from build123d import *

# Parameters (mm, degrees)
BOSS_EXTRUDE1_DEPTH  = 5
CUT_EXTRUDE1_DEPTH   = 10
BOSS_EXTRUDE3_START  = -3
SKETCH13_R           = 2.5
BOSS_EXTRUDE3_DEPTH  = 3
CHAMFER1_SIZE        = 2
BOSS_EXTRUDE7_DEPTH  = 17
SKETCH22_R           = 1.6
CUT_EXTRUDE4_DEPTH   = 20
CUT_EXTRUDE5_DEPTH   = 7
BOSS_EXTRUDE8_START  = -20
BOSS_EXTRUDE8_DEPTH  = 20
SKETCH26_R           = 90.5
SKETCH26_R_2         = 90
CUT_EXTRUDE6_DEPTH   = 15
BOSS_EXTRUDE9_START  = 20
BOSS_EXTRUDE9_DEPTH  = 20
BOSS_EXTRUDE11_DEPTH = 20
FILLET2_R            = 6
CUT_EXTRUDE8_DEPTH   = 5
FILLET3_R            = 5
CUT_EXTRUDE9_DEPTH   = 5
FILLET4_R            = 3
CUT_EXTRUDE11_DEPTH  = 5
FILLET5_R            = 3


# Some blends are built 0.0001 mm under size
with BuildPart() as part:
    # Sketch1 → Boss-Extrude1 (new body)
    with BuildSketch(Plane.XY):
        with BuildLine():
            Line((10, 70), (0, 70))
            Line((0, 70), (0, 40))
            ThreePointArc((0, 40), (34.641016151, 20), (34.641016151, -20))
            Line((34.641016151, -20), (50.226140717, -28.998075863))
            ThreePointArc((50.226140717, -28.998075863), (74.464134482, -30.098388714), (89.334294573, -10.926290001))
            ThreePointArc((89.334294573, -10.926290001), (70.606727842, 55.809407661), (10, 89.4427191))
            Line((10, 89.4427191), (10, 70))
        make_face()
    extrude(amount=-BOSS_EXTRUDE1_DEPTH)

    # Sketch10 → Cut-Extrude1 (cut)
    with BuildSketch(Plane.ZY):
        Polygon((-5, 70), (0, 47.166644618), (0, 70), align=None)
    extrude(amount=-CUT_EXTRUDE1_DEPTH, mode=Mode.SUBTRACT)

    # Sketch13 → Boss-Extrude3 (add)
    # profile 1 of 2: a face of its own
    with BuildSketch(Plane.XY.offset(BOSS_EXTRUDE3_START)):
        with BuildLine():
            Line((37.380217316, 94.74443559), (31.380217316, 84.352130745))
            ThreePointArc((31.380217316, 84.352130745), (45, 77.942286341), (57.36097943, 69.352130745))
            Line((57.36097943, 69.352130745), (63.36097943, 79.74443559))
            Line((63.36097943, 79.74443559), (37.380217316, 94.74443559))
        make_face()
        with Locations((40.856551784, 85.765623512)):
            Circle(SKETCH13_R, mode=Mode.SUBTRACT)
        with Locations((53.846932841, 78.265623512)):
            Circle(SKETCH13_R, mode=Mode.SUBTRACT)
    # profile 2 of 2: a face of its own
    with BuildSketch(Plane.XY.offset(BOSS_EXTRUDE3_START)):
        with BuildLine():
            Line((79.611529559, 63.493885461), (69.234612109, 57.502769378))
            ThreePointArc((69.234612109, 57.502769378), (77.850059036, 45.159365674), (84.287765503, 31.552695391))
            Line((84.287765503, 31.552695391), (94.611529559, 37.513123348))
            Line((94.611529559, 37.513123348), (79.611529559, 63.493885461))
        make_face()
        with Locations((85.63271748, 40.989457815)):
            Circle(SKETCH13_R, mode=Mode.SUBTRACT)
        with Locations((78.13271748, 53.979838872)):
            Circle(SKETCH13_R, mode=Mode.SUBTRACT)
    extrude(amount=BOSS_EXTRUDE3_DEPTH)

    # Chamfer1
    chamfer1_edges = [part.edges().sort_by_distance(p)[0] for p in [
        (45, 77.942286341, -3),
    ]]
    chamfer(chamfer1_edges, length=CHAMFER1_SIZE - 0.0001)  # a hair under: the kernel refuses the full size

    # Sketch21 → Boss-Extrude7 (add)
    with BuildSketch(Plane(origin=(0, 0, -3), x_dir=(-1, 0, 0), z_dir=(0, 0, -1))):
        with BuildLine():
            Line((-32.394087652, 86.108205679), (-37.380217316, 94.74443559))
            Line((-37.380217316, 94.74443559), (-63.36097943, 79.74443559))
            Line((-63.36097943, 79.74443559), (-58.374849766, 71.108205679))
            ThreePointArc((-58.374849766, 71.108205679), (-46, 79.674337148), (-32.394087652, 86.108205679))
        make_face()
        with BuildLine():
            Line((-86.043250616, 32.566225194), (-94.611529559, 37.513123348))
            Line((-94.611529559, 37.513123348), (-79.611529559, 63.493885461))
            Line((-79.611529559, 63.493885461), (-70.991284652, 58.516984744))
            ThreePointArc((-70.991284652, 58.516984744), (-79.582170095, 46.159269957), (-86.043250616, 32.566225194))
        make_face()
    extrude(amount=BOSS_EXTRUDE7_DEPTH)

    # Sketch22 → Cut-Extrude4 (cut)
    with BuildSketch(Plane.XY):
        with Locations(Location((40.856551784, 85.765623512, 0), (0, 0, 180))):
            Circle(SKETCH22_R)
        with Locations(Location((53.846932841, 78.265623512, 0), (0, 0, 180))):
            Circle(SKETCH22_R)
        with Locations(Location((78.13271748, 53.979838872, 0), (0, 0, 180))):
            Circle(SKETCH22_R)
        with Locations(Location((85.63271748, 40.989457815, 0), (0, 0, 180))):
            Circle(SKETCH22_R)
    extrude(amount=-CUT_EXTRUDE4_DEPTH, mode=Mode.SUBTRACT)

    # Sketch24 → Cut-Extrude5 (cut)
    with BuildSketch(Plane.XY):
        Polygon((42.741480602, 83.428878621), (43.82269663, 86.229647308), (41.937767812, 88.566392198), (38.971622965, 88.102368402), (37.890406937, 85.301599716), (39.775335756, 82.964854825), align=None)
        Polygon((55.059031292, 75.518961778), (56.831660903, 77.942000695), (55.619562452, 80.688662429), (52.634834389, 81.012285245), (50.862204778, 78.589246328), (52.074303229, 75.842584594), align=None)
        Polygon((78.97688632, 51.098743194), (81.049903948, 53.270362694), (80.205735108, 56.151458371), (77.28854864, 56.860934549), (75.215531013, 54.68931505), (76.059699853, 51.808219373), align=None)
        Polygon((86.409892613, 38.089572965), (88.532678995, 40.212568798), (87.755503862, 43.112453649), (84.855542347, 43.889342666), (82.732755965, 41.766346832), (83.509931098, 38.866461981), align=None)
    extrude(amount=-CUT_EXTRUDE5_DEPTH, mode=Mode.SUBTRACT)

    # Sketch25 → Boss-Extrude8 (add)
    with BuildSketch(Plane(origin=(0, 0, -20), x_dir=(-1, 0, 0), z_dir=(0, 0, -1)).offset(BOSS_EXTRUDE8_START)):
        with BuildLine():
            Line((-86.043250616, 32.566225194), (-84.287765503, 31.552695391))
            ThreePointArc((-84.287765503, 31.552695391), (-77.850059036, 45.159365674), (-69.234612109, 57.502769378))
            Line((-69.234612109, 57.502769378), (-70.991284652, 58.516984744))
            ThreePointArc((-70.991284652, 58.516984744), (-79.582170095, 46.159269957), (-86.043250616, 32.566225194))
        make_face()
        with BuildLine():
            Line((-58.374849766, 71.108205679), (-57.36097943, 69.352130745))
            ThreePointArc((-57.36097943, 69.352130745), (-45, 77.942286341), (-31.380217316, 84.352130745))
            Line((-31.380217316, 84.352130745), (-32.394087652, 86.108205679))
            ThreePointArc((-32.394087652, 86.108205679), (-46, 79.674337148), (-58.374849766, 71.108205679))
        make_face()
    extrude(amount=BOSS_EXTRUDE8_DEPTH)

    # Sketch26 → Cut-Extrude6 (cut)
    with BuildSketch(Plane(origin=(0, 0, -5), x_dir=(-1, 0, 0), z_dir=(0, 0, -1))):
        Circle(SKETCH26_R)
        Circle(SKETCH26_R_2, mode=Mode.SUBTRACT)
    extrude(amount=CUT_EXTRUDE6_DEPTH, mode=Mode.SUBTRACT)

    # Sketch28 → Boss-Extrude9 (add)
    with BuildSketch(Plane.XY.offset(BOSS_EXTRUDE9_START)):
        with BuildLine():
            Line((23.533293218, 36.154783936), (43.701329204, 19.231792379))
            Line((43.701329204, 19.231792379), (40, 0))
            ThreePointArc((40, 0), (33.797136862, 21.395175623), (17.112323002, 36.154783936))
            Line((17.112323002, 36.154783936), (23.533293218, 36.154783936))
        make_face()
    extrude(amount=-BOSS_EXTRUDE9_DEPTH)

    # Sketch30 → Boss-Extrude11 (add)
    with BuildSketch(Plane.XY):
        with BuildLine():
            Line((31.380217316, 84.352130745), (37.380217316, 94.74443559))
            ThreePointArc((37.380217316, 94.74443559), (-25.433217284, 98.625251232), (-78.536554117, 64.8521271))
            Line((-78.536554117, 64.8521271), (-69.397791898, 57.305728157))
            ThreePointArc((-69.397791898, 57.305728157), (-23.328329719, 86.92404174), (31.380217316, 84.352130745))
        make_face()
    extrude(amount=-BOSS_EXTRUDE11_DEPTH)

    # Fillet2
    # the kernel refuses this fillet: 6 mm, written as the material it takes off along each edge
    with BuildSketch(Plane(origin=(-69.397791898, 57.305728157, 14.53079134), x_dir=(0.6605272706079757, 0.7508020543280219, 0), z_dir=(0, 0, -1))) as fillet2_piece_1:
        with BuildLine():
            CenterArc((5.815342996, -5.997066729), FILLET2_R, 91.791660849, 86.416678302)
            Line((-0.181723733, -5.809475019), (0, 0))
            ThreePointArc((0, 0), (2.813875643, -0.043999067), (5.627751287, 0))
        make_face()
    extrude(amount=49.06158268, mode=Mode.SUBTRACT)
    with BuildSketch(Plane(origin=(-78.536554117, 64.8521271, 15.946769714), x_dir=(0.6605636178718797, 0.7507700758181651, 0), z_dir=(0, 0, -1))) as fillet2_piece_2:
        with BuildLine():
            CenterArc((6.190825845, 5.99705764), FILLET2_R, 178.205565332, 93.588869337)
            Line((0.193768204, 6.184939681), (0, 0))
            ThreePointArc((0, 0), (3.189353943, -0.049947441), (6.378707886, 0))
        make_face()
    extrude(amount=51.893539428, mode=Mode.SUBTRACT)

    # Sketch31 → Cut-Extrude8 (cut)
    with BuildSketch(Plane(origin=(0, 0, 0), x_dir=(-1, 0, 0), z_dir=(0, 0, -1))):
        Polygon((-126.538851056, -27.990413584), (-128.420531953, -25.747913615), (-227.900156191, -109.221229623), (-215.044403998, -124.542118485), (-23.533293218, 36.154783936), (-24.818868437, 37.686872822), (-88.130475533, 4.238040152), align=None)
    extrude(amount=CUT_EXTRUDE8_DEPTH, mode=Mode.SUBTRACT)

    # Fillet3
    fillet3_edges = [part.edges().sort_by_distance(p)[0] for p in [
        (87.283893388, -17.338321154, -2.5),
    ]]
    fillet(fillet3_edges, radius=FILLET3_R)

    # Sketch32 → Cut-Extrude9 (cut)
    with BuildSketch(Plane.XY):
        Polygon((87.46553992, 4.589339402), (92.809930085, 1.765787441), (89.670227424, 2.292669877), align=None)
    extrude(amount=-CUT_EXTRUDE9_DEPTH, mode=Mode.SUBTRACT)

    # Fillet4
    fillet4_edges = [part.edges().sort_by_distance(p)[0] for p in [
        (89.94013986, 3.281957025, -2.5),
    ]]
    fillet(fillet4_edges, radius=FILLET4_R)

    # Sketch33 → Cut-Extrude11 (cut)
    with BuildSketch(Plane.XY):
        Polygon((24.818868437, 37.686872822), (88.601440511, 3.989219605), (89.06857455, 4.873406118), (25.286002476, 38.571059335), align=None)
    extrude(amount=-CUT_EXTRUDE11_DEPTH, mode=Mode.SUBTRACT)

    # Fillet5
    # the kernel refuses this fillet: 3 mm, written as the material it takes off along each edge
    with BuildSketch(Plane(origin=(87.631958407, 5.632400166, -16.76496935), x_dir=(0.385373580220951, 0.9227606426737577, 0), z_dir=(0, 0, 1))) as fillet5_piece_1:
        with BuildLine():
            CenterArc((3.250174857, 2.623091468), FILLET5_R, 174.818513503, 124.211713056)
            Line((0.262433961, 2.894023819), (-0.036340129, 2.921117054))
            Line((-0.036340129, 2.921117054), (-0.29877409, 0.027093235))
            Line((-0.29877409, 0.027093235), (-0.219376832, -0.204630901))
            ThreePointArc((-0.219376832, -0.204630901), (3.755091894, -0.860969557), (4.851569028, -0.262309147))
            Line((4.851569028, -0.262309147), (4.70598774, 0))
        make_face()
    extrude(amount=28.529938699, mode=Mode.SUBTRACT)


solid = part.part
Input: part model. Units: mm. Frame: model coordinates. A direction names the side the tool comes from. Coordinates: 2 decimals unless noted, no trailing zeros. Write each loop counter-clockwise with the first axis right and the second up, starting at its lowest first coordinate (ties: lowest second). Pieces come first, ordered by that corner, then holes. Notation, with made-up numbers: M 79.25,-19.5 L 132.25,-19.5 A21 cw 132.25,3.5 Z; hole C 30.25,20 d11. An arc over 180 degrees is marked long. Answer as a JSON object with one key per item and string values. Group by question number.
(1) Ray query, line 1 along Z through (x, y) = (48, 62); line 2 along Z through (x, y) = (-2.5, 92); line 3 along Y through (x, z) = (0, -12). Return the intervals inside material, ascending. Write a range as [from, to].
(2) Section B-B on y = 23. Output: boundary loops of the cut face in (x, z).
(3) Contact query for flat-ended pins moving along their axis: P1, Ø6, axis at y = 35.5, z = 1, coming from the +X side; P2, Ø7, axis at x = 20.5, z = 7.5, coming from the +Y side; P3, Ø3, axis at x = 40.5, y = 85, coming from the +Z side; P4, Ø1.5, axis at x = 76, y = 49.5, coming from the +Z side. Output: stop coordinate, or through.
(4) Mould query, pull axis Y, two halves, no side actions, for faces 1 (the face through (82, 48, -20)), 2 (the face through (4.93, 58.743, -2.535)), 3 (the face through (41.877, 9.751, 10.14)). Classes: pulls with the +Y half, pulls with the -Y half, needs draft (parallel to the pull), parting line crosses it, or undercut.
(5) Section D-D on x = 21.5. Output: boundary loops of the cut face in (y, z), plus the area to 3 significant figures.
(6) Set-up query: faces 4 (the face through (45.07, 78.48, -12.4)), 5 (the face through (87.57, 20.77, -2.46)), 6 (the face through (27, 65, 0)), 7 (the face through (79.4, 52.7, -7)), 8 (the face through (0, 52, -3)). Return all of +Z, -Z, +X, -X, +Y, -Y with unobstructed straight access to the full face (end or side cutting, diameter ignored); none if empty.
(7) Section A-A on z = -11.5. Output: boundary loops of the cut face in (x, y), plus the area to 3 significant figures.
(8) Section C-C on x = 3. Output: boundary loops of the cut face in (y, z), plus the area to 3 significant figures.
Result set:
{
 "1": {"line 1": "z = [-5, 0]", "line 2": "z = [-20, 0]", "line 3": "y = [90, 101.85]"},
 "2": {"outline": "M 32.73,-5 L 39.21,-5 L 39.21,20 L 32.73,20 Z; M 54.76,-5 L 87.01,-5 L 87.01,0 L 54.76,0 Z"},
 "3": {"P1": "stops at x = 94.61", "P2": "stops at y = 36.15", "P3": "stops at z = -7", "P4": "stops at z = 0"},
 "4": {"face 1": "needs draft", "face 2": "undercut", "face 3": "pulls with the -Y half"},
 "5": {"outline": "M 33.73,-5 L 87.39,-5 L 87.39,-20 L 99.56,-20 L 99.56,0 L 36.15,0 L 36.15,20 L 33.73,20 Z", "area": "560 mm2"},
 "6": {"face 4": "-Z, -Y", "face 5": "+Z, -Z, +X", "face 6": "+Z, +X, +Y", "face 7": "+Z", "face 8": "+Z, -Z, -Y"},
 "7": {"outline": "M -74.32,69.64 A6 ccw -73.82,60.96 A6 ccw -65.68,61.53 A90 cw 31.38,84.35 L 31.63,84.79 A90.5 cw 57.61,69.79 L 63.36,79.74 L 37.38,94.74 A101.85 ccw Z; M 69.67,57.76 A90.5 cw 84.73,31.81 L 94.61,37.51 L 79.61,63.49 Z; hole C 40.86,85.77 d3.2; hole C 53.85,78.27 d3.2; hole C 78.13,53.98 d3.2; hole C 85.63,40.99 d3.2", "area": "2,010 mm2"},
 "8": {"outline": "M 39.89,-5 L 70,-5 L 47.17,0 L 39.89,0 Z; M 89.95,-20 L 101.81,-20 L 101.81,0 L 89.95,0 Z", "area": "331 mm2"}
}
